from build123d import *

# Parameters (mm, degrees)
SKIZZE2_R                       = 4.5
AUFSATZ_LINEAR_AUSTRAGEN1_DEPTH = 12
SCHNITT_LINEAR_AUSTRAGEN6_DEPTH = 5
SCHNITT_LINEAR_AUSTRAGEN1_DEPTH = 62.290292869
SCHNITT_LINEAR_AUSTRAGEN5_DEPTH = 62.290292869
SKIZZE6_W                       = 18
SKIZZE6_H                       = 25
SCHNITT_LINEAR_AUSTRAGEN7_DEPTH = 6
AUFSATZ_LINEAR_AUSTRAGEN2_DEPTH = 3
AUFSATZ_LINEAR_AUSTRAGEN3_DEPTH = 3
SCHNITT_LINEAR_AUSTRAGEN8_DEPTH = 62.290292869
FASE1_SIZE                      = 10


with BuildPart() as part:
    # Skizze2 → Aufsatz-Linear austragen1 (new body)
    with BuildSketch(Plane.XY):
        with BuildLine():
            Line((-7.5, 42.5), (-7.5, 24.5))
            Line((-7.5, 24.5), (17.5, 24.5))
            ThreePointArc((17.5, 24.5), (22.449747468, 22.449747468), (24.5, 17.5))
            Line((24.5, 17.5), (24.5, -7.5))
            Line((24.5, -7.5), (42.5, -7.5))
            Line((42.5, -7.5), (42.5, 42.5))
            Line((42.5, 42.5), (-7.5, 42.5))
        make_face()
        with Locations((33.5, 33.5)):
            Circle(SKIZZE2_R, mode=Mode.SUBTRACT)
    extrude(amount=AUFSATZ_LINEAR_AUSTRAGEN1_DEPTH)

    # Skizze5 → Schnitt-Linear austragen6 (cut)
    with BuildSketch(Plane.XY.offset(12)):
        Polygon((41.005553499, 33.5), (37.25277675, 40), (29.74722325, 40), (25.994446501, 33.5), (29.74722325, 27), (37.25277675, 27), align=None)
    extrude(amount=-SCHNITT_LINEAR_AUSTRAGEN6_DEPTH, mode=Mode.SUBTRACT)

    # Skizze3 → Schnitt-Linear austragen1 (cut, through all)
    with BuildSketch(Plane(origin=(0, 0, 0), x_dir=(1, 0, 0), z_dir=(0, 1, 0))):
        with BuildLine():
            Line((3, 4.576951254), (3, -0.5))
            ThreePointArc((3, -0.5), (0, -3.5), (-3, -0.5))
            Line((-3, -0.5), (-3, 4.576951254))
            ThreePointArc((-3, 4.576951254), (0, 7.576951254), (3, 4.576951254))
        make_face()
    extrude(amount=SCHNITT_LINEAR_AUSTRAGEN1_DEPTH, mode=Mode.SUBTRACT)

    # Skizze4 → Schnitt-Linear austragen5 (cut, through all)
    with BuildSketch(Plane(origin=(0, 0, 0), x_dir=(0, 0, -1), z_dir=(1, 0, 0))):
        with BuildLine():
            Line((-0.5, -3), (-6.5, -3))
            ThreePointArc((-6.5, -3), (-9.5, 0), (-6.5, 3))
            Line((-6.5, 3), (-0.5, 3))
            ThreePointArc((-0.5, 3), (2.5, 0), (-0.5, -3))
        make_face()
    extrude(amount=SCHNITT_LINEAR_AUSTRAGEN5_DEPTH, mode=Mode.SUBTRACT)

    # Skizze6 → Schnitt-Linear austragen7 (cut)
    with BuildSketch(Plane(origin=(0, 0, 0), x_dir=(-1, 0, 0), z_dir=(0, 0, -1))):
        with Locations((-33.5, 5)):
            Rectangle(SKIZZE6_W, SKIZZE6_H)
    extrude(amount=-SCHNITT_LINEAR_AUSTRAGEN7_DEPTH, mode=Mode.SUBTRACT)

    # Skizze7 → Aufsatz-Linear austragen2 (add)
    with BuildSketch(Plane(origin=(42.5, 0, 0), x_dir=(0, 0, -1), z_dir=(1, 0, 0))):
        Polygon((-6, 3), (-6, 17.5), (0, 17.5), align=None)
    extrude(amount=-AUFSATZ_LINEAR_AUSTRAGEN2_DEPTH)

    # Skizze8 → Aufsatz-Linear austragen3 (add)
    with BuildSketch(Plane.ZY.offset(-24.5)):
        Polygon((6, 3), (6, 17.5), (0, 17.5), align=None)
    extrude(amount=-AUFSATZ_LINEAR_AUSTRAGEN3_DEPTH)

    # Skizze9 → Schnitt-Linear austragen8 (cut, through all)
    with BuildSketch(Plane(origin=(0, 0, 0), x_dir=(-1, 0, 0), z_dir=(0, 0, -1))):
        with BuildLine():
            Line((-18.5, 39.5), (-10, 39.5))
            ThreePointArc((-10, 39.5), (-4, 33.5), (-10, 27.5))
            Line((-10, 27.5), (-18.5, 27.5))
            ThreePointArc((-18.5, 27.5), (-24.5, 33.5), (-18.5, 39.5))
        make_face()
    extrude(amount=-SCHNITT_LINEAR_AUSTRAGEN8_DEPTH, mode=Mode.SUBTRACT)

    # Fase1
    fase1_edges = [part.edges().sort_by_distance(p)[0] for p in [
        (-7.5, 33.5, 12),
    ]]
    chamfer(fase1_edges, length=FASE1_SIZE)


solid = part.part
Work out the finished part from the listing and answer in its coordinate system (mm). A direction names the side the tool comes from. Give positions to 0.01 mm unless a question says otherwise; leave off trailing zeros. Loops run counter-clockwise (first coordinate to the right, second up) from the corner with the lowest first, then second, coordinate; pieces in that order, holes last. Notation, with made-up numbers: (74.25, 16.5) -> (96.25, 16.5) arc R19 cw to (96.25, 40.5) -> close; hole circle Ø1 at (27, -10). An arc over 180 degrees is marked (long way). Use a Markdown table: item, result. Add a question column.
1) Each of these flat-tipped pins is pushed along its axis until it touches: P1, Ø2.5, axis at x = 16, z = 6, coming from the -Y side; P2, Ø4, axis at x = 20.5, z = 5.5, coming from the -Y side; P3, Ø1.8, axis at x = 34, z = 2, coming from the -Y side. Where does it stop, or does it pass through?
2) Consider line 1 along Y through (x, z) = (11.5, 2.5); line 2 along Y through (x, z) = (33.5, 2.5); line 3 along X through (y, z) = (33.5, 2.5). Determine where each line is inside the solid, lowest interval first.
3) Which of the six approach directions +Z, -Z, +X, -X, +Y, -Y give full straight-line access (tool end or side, diameter ignored) to faces 1 (the flat face through (39.5, 14, 4)), 2 (the flat face through (35, 38, 7)), 3 (the flat face through (24.5, 8, 7)), 4 (the flat face through (14, 27.5, 6))?
4) The part is cut by section D-D, the plane x = 21. Determine the outline of the cut face in (y, z).
5) The part is cut by section B-B, the plane z = 8. Determine the outline of the cut face in (x, y).
6) For a pull along Y with two mould halves and no side action, classify faces 5 (the cylindrical face through (24.5, 33.4, 5.9)), 6 (the flat face through (18, 42.5, 6)), 7 (the flat face through (25.98, 10.35, 2.96)), 8 (the flat face through (31, 18, 12)) as +Y half, -Y half, draft (parallel to the pull), parting line (faces both ways), or undercut.
7) The part is cut by section A-A, the plane x = 33.5. Determine the outline of the cut face in (y, z).
8) The part is cut by section C-C, the plane y = 4. Determine the outline of the cut face in (x, z), plus the area to 3 significant figures.
Reported:
| question | item | result |
|---|---|---|
| 1 | P1 | stops at y = 24.5 |
| 1 | P2 | stops at y = 22.4 |
| 1 | P3 | stops at y = 17.5 |
| 2 | line 1 | y = 24.5 to 27.5, 39.5 to 42.5 |
| 2 | line 2 | y = 17.5 to 29, 38 to 42.5 |
| 2 | line 3 | x = -7 to -2.24, 2.24 to 4, 24.5 to 29, 38 to 42.5 |
| 3 | face 1 | -Z, -Y |
| 3 | face 2 | +Z |
| 3 | face 3 | +Z, -Z, -X, -Y |
| 3 | face 4 | +Z, -Z |
| 4 | outline | (23.56, 0) -> (28.05, 0) -> (28.05, 12) -> (23.56, 12) -> close; (38.95, 0) -> (42.5, 0) -> (42.5, 12) -> (38.95, 12) -> close |
| 5 | outline | (-1.5, 24.5) -> (17.5, 24.5) arc R7 cw to (24.5, 17.5) -> (24.5, 2.6) -> (42.5, 2.6) -> (42.5, 42.5) -> (-1.5, 42.5) -> close; (24.5, -7.5) -> (42.5, -7.5) -> (42.5, -2.6) -> (24.5, -2.6) -> close; hole (10, 27.5) -> (18.5, 27.5) arc R6 ccw to (18.5, 39.5) -> (10, 39.5) arc R6 ccw to start; hole (25.99, 33.5) -> (29.75, 27) -> (37.25, 27) -> (41.01, 33.5) -> (37.25, 40) -> (29.75, 40) -> close |
| 6 | face 5 | undercut |
| 6 | face 6 | +Y half |
| 6 | face 7 | -Y half |
| 6 | face 8 | draft |
| 7 | outline | (-7.5, 6) -> (-3, 6) -> (-3, 6.5) arc R3 cw to (3, 6.5) -> (3, 6) -> (17.5, 6) -> (17.5, 0) -> (29, 0) -> (29, 7) -> (27, 7) -> (27, 12) -> (-7.5, 12) -> close; (38, 0) -> (42.5, 0) -> (42.5, 12) -> (40, 12) -> (40, 7) -> (38, 7) -> close |
| 8 | outline | (24.5, 5.59) -> (27.5, 5.59) -> (27.5, 6) -> (39.5, 6) -> (39.5, 5.59) -> (42.5, 5.59) -> (42.5, 12) -> (24.5, 12) -> close |
| 8 | area | 110 mm^2 |
